Verification items for the finished model (mm, model axes). Round coordinates to 2 decimals unless told otherwise and drop trailing zeros. Write each loop counter-clockwise with the first axis right and the second up, starting at its lowest first coordinate (ties: lowest second). Pieces come first, ordered by that corner, then holes.
from build123d import *

# Parameters (mm, degrees)
SKETCH1_W           = 279.4
SKETCH1_H           = 279.4
BOSS_EXTRUDE1_DEPTH = 5.9944
SKETCH2_R           = 7.25
CUT_EXTRUDE1_DEPTH  = 198.656552715
FILLET1_R           = 2.54
SKETCH3_R           = 1
CUT_EXTRUDE2_DEPTH  = 198.656552715


with BuildPart() as part:
    # Sketch1 → Boss-Extrude1 (new body)
    with BuildSketch(Plane(origin=(0, 0, 0), x_dir=(1, 0, 0), z_dir=(0, 1, 0))):
        Rectangle(SKETCH1_W, SKETCH1_H)
    extrude(amount=BOSS_EXTRUDE1_DEPTH)

    # Sketch2 → Cut-Extrude1 (cut, through all)
    with BuildSketch(Plane(origin=(0, 5.9944, 0), x_dir=(1, 0, 0), z_dir=(0, 1, 0))):
        with Locations(Location((-63.5, 63.5, 0), (0, 0, 270))):
            Circle(SKETCH2_R)
        with Locations(Location((63.5, 63.5, 0), (0, 0, 270))):
            Circle(SKETCH2_R)
        with Locations(Location((63.5, -63.5, 0), (0, 0, 270))):
            Circle(SKETCH2_R)
        with Locations(Location((-63.5, -63.5, 0), (0, 0, 270))):
            Circle(SKETCH2_R)
    extrude(amount=-CUT_EXTRUDE1_DEPTH, mode=Mode.SUBTRACT)

    # Fillet1
    fillet1_edges = [part.edges().sort_by_distance(p)[0] for p in [
        (139.7, 2.9972, 139.7),
        (-139.7, 2.9972, 139.7),
        (-139.7, 2.9972, -139.7),
        (139.7, 2.9972, -139.7),
    ]]
    fillet(fillet1_edges, radius=FILLET1_R)

    # Sketch3 → Cut-Extrude2 (cut, through all)
    with BuildSketch(Plane(origin=(0, 5.9944, 0), x_dir=(1, 0, 0), z_dir=(0, 1, 0))):
        with BuildLine():
            ThreePointArc((2.5, 124.7), (0, 127.2), (-2.5, 124.7))
            Line((-2.5, 124.7), (2.5, 124.7))
        make_face()
        with BuildLine():
            Line((2.5, 124.7), (-2.5, 124.7))
            ThreePointArc((-2.5, 124.7), (0, 122.2), (2.5, 124.7))
        make_face()
        with Locations(Location((7.5, 124.7, 0), (0, 0, 270))):
            Circle(SKETCH3_R)
        with Locations(Location((-7.5, 124.7, 0), (0, 0, 270))):
            Circle(SKETCH3_R)
    extrude(amount=-CUT_EXTRUDE2_DEPTH, mode=Mode.SUBTRACT)


solid = part.part
Q1. Material ranges on line 1 along X through (y, z) = (2.1, -63.5); line 2 along Z through (x, y) = (59, 2.95); line 3 along Z through (x, y) = (-62, 1.7), recorded low to high.
Recorded:
line 1: x = -139.7 to -70.75, -56.25 to 56.25, 70.75 to 139.7
line 2: z = -139.7 to -69.18, -57.82 to 57.82, 69.18 to 139.7
line 3: z = -139.7 to -70.59, -56.41 to 56.41, 70.59 to 139.7
Q2. Sectioned sample at B-B (z = -63.5). Enter the section's corners in (x, y).
Recorded:
outline: (-139.7, 0) - (-70.75, 0) - (-70.75, 5.99) - (-139.7, 5.99) - close; (-56.25, 0) - (56.25, 0) - (56.25, 5.99) - (-56.25, 5.99) - close; (70.75, 0) - (139.7, 0) - (139.7, 5.99) - (70.75, 5.99) - close
Q3. Release check for a two-part mould opening along X. For faces 1 (the cylindrical face through (59.088, 3.039, 57.747)), 2 (the flat face through (139.7, 3, 2)), 3 (the flat face through (-2, 0, -2)), 4 (the cylindrical face through (-67.912, 3.039, 57.747)) record: released by +X, released by -X, zero draft, split by the parting line, or undercut.
Recorded:
face 1: undercut
face 2: released by +X
face 3: zero draft
face 4: undercut
Q4. Sectioned sample at A-A (x = 63.5). Enter the section's corners in (y, z), plus the area to 3 significant figures.
Recorded:
outline: (0, -139.7) - (5.99, -139.7) - (5.99, -70.75) - (0, -70.75) - close; (0, -56.25) - (5.99, -56.25) - (5.99, 56.25) - (0, 56.25) - close; (0, 70.75) - (5.99, 70.75) - (5.99, 139.7) - (0, 139.7) - close
area: 1,500 mm2
